Autodesk Inventor part; units mm, degrees
ref_plane "YZ Plane" through (0, 0, 0) normal (1, 0, 0) x (0, 1, 0)
ref_plane "XZ Plane" through (0, 0, 0) normal (0, 1, 0) x (-1, 0, 0)
ref_plane "XY Plane" through (0, 0, 0) normal (0, 0, 1) x (1, 0, 0)
sketch "Sketch1" plane through (0, 0, 0) normal (1, 0, 0) x (0, 1, 0)
  line L0 (0, -4.8819) -> (5, -4.8819)
  line L1 (5, -4.8819) -> (0, -4.8819)
  line L2 (0, -4.8819) -> (0, -9.8819)
  line L3 (0, -9.8819) -> (5, -9.8819)
  arc A0 (15, -4.8819) -> (5, -4.8819) centre (10, -8.1985) ccw
  arc A1 (5, -9.8819) -> (15, -9.8819) centre (10, -6.5653) ccw
  line L4 (15, -9.8819) -> (15, -4.8819)
  point P0 (0, 0)
  point P1 (0, -7.3819)
  point P2 (10, -7.3819)
  point P3 (10, -4.8819)
  point P4 (10, -9.8819)
  dimension "d0" = 5
  dimension "d1" = 10
  dimension "d2" = 5
  dimension "d3" = 5
  dimension "d4" = 10
  dimension "d5" = 6
  dimension "d6" = 6
extrude "Extrusion1" add sketch "Sketch1" along normal blind 10
sketch "Sketch7" plane through (10, 0, 0) normal (1, 0, 0) x (0, 0, -1)
  line L0 (9.8819, 15) -> (4.8819, 15)
  line L1 (9.8819, 0) -> (9.8819, 5)
  line L2 (4.8819, 0) -> (9.8819, 0)
  circle A0 centre (7.3819, 9) radius 4
  point P0 (0, 0)
  point P1 (7.3819, 15)
  point P2 (7.3819, 5)
  point P3 (9.8819, 10.0351)
  dimension "d29" = 2.5
  dimension "d30" = 10
  dimension "d31" = 4
  dimension "d33" = 5
extrude "Extrusion4" cut sketch "Sketch7" against normal blind 10
sketch "Sketch8" plane through (10, 0, 0) normal (1, 0, 0) x (0, 0, -1)
  line L0 (8.3819, 12.873) -> (8.3819, 15)
  line L1 (9.8819, 15) -> (4.8819, 15)
  line L2 (9.8819, 15) -> (4.8819, 15)
  line L3 (6.3819, 15) -> (6.3819, 12.873)
  circle A0 centre (7.3819, 9) radius 4
  line L4 (8.3819, 15) -> (6.3819, 15)
  arc A1 (8.3819, 12.873) -> (6.3819, 12.873) centre (7.3819, 9) ccw
  point P0 (0, 0)
  dimension "d36" = 1.5
  dimension "d39" = 1.5
extrude "Extrusion5" cut sketch "Sketch8" against normal blind 10 contours A0 L3 L1 L0
sketch "Sketch9" plane through (0, 0, -9.8819) normal (0, 0, -1) x (-1, 0, 0)
  circle A0 centre (-5, 13.9365) radius 0.4
  line L0 (-10, 12.873) -> (0, 12.873)
  line L1 (0, 15) -> (-10, 15)
  line L2 (-10, 15) -> (-10, 5)
  point P0 (0, 0)
  dimension "d42" = 0.8
  dimension "d43" = 1.0635
  dimension "d44" = 2.127
  dimension "d45" = 10
  dimension "d46" = 5
hole "Hole1" at (5, 13.9365, -9.8819) direction (0, 0, -1) diameter 1.5 end through all both
sketch "Sketch10" plane through (0, 0, -9.8819) normal (0, -1, 0) x (1, 0, 0)
  line L0 (12, -2) -> (12, 7)
  line L1 (12, 7) -> (-2, 7)
  line L2 (0, 7.6834) -> (10, 7.6834)
  line L3 (-2, 7) -> (-2, -2)
  line L4 (-2, -2) -> (12, -2)
  line L5 (0, -2.6834) -> (10, -2.6834)
  line L6 (0, -2.6834) -> (0, 0)
  line L7 (0, 0) -> (10, 0)
  line L8 (0, 5) -> (0, 0)
  line L9 (0, 5) -> (10, 5)
  point P0 (0, 9.8819)
  point P1 (5, 2.5)
  dimension "d54" = 14
  dimension "d56" = 2
  dimension "d57" = 2
  dimension "d58" = 5
  dimension "d59" = 2.5
  dimension "d60" = 2
  dimension "d74" = 9
extrude "Extrusion6" add sketch "Sketch10" along normal blind 1.5
sketch "Sketch11" plane through (10, 0, 0) normal (1, 0, 0) x (0, 0, -1)
  point P0 (0, 0)
sketch "Sketch12" plane through (0, -1.5, -9.8819) normal (0, -1, 0) x (1, 0, 0)
  line L0 (-2, 7) -> (-2, -2)
  line L1 (12, 7) -> (-2, 7)
  circle A0 centre (5, 2.5) radius 2.5
  point P0 (0, 9.8819)
  dimension "d63" = 7
  dimension "d64" = 4.5
  dimension "d65" = 9
  dimension "d66" = 5
hole "Hole2" at (5, -1.5, -7.3819) direction (0, 1, 0) diameter 5 depth 1.5
equation "\"d2\" = d0"
equation "\"d3\" = d0"
equation "\"d36\" = d37"
equation "\"d43\" = 0.5 * d44"
equation "\"d60\" = d57"
equation "\"d66\" = hoop_bearing_length"
equation "\"hoop_bearing_length\" = 5"
properties part number "Clamp"
The model under review builds one solid part; all positions refer to its coordinate system, in mm. A direction names the side the tool comes from. Round coordinates to 2 decimals unless told otherwise and drop trailing zeros. Order: outer loops, then holes, each group sorted by start corner. A loop starts at its lowest first (then second) coordinate and runs counter-clockwise, first axis right, second up. Notation, with made-up numbers: M -9.5,41 L 27.5,41 A27 ccw 27.5,68 Z; hole C 4.25,62.5 d10. An arc over 180 degrees is marked long. Use a Markdown table: item, result.
1) Tool access review of faces 4 (the face through (6, 14, -6.382)), 5 (the face through (10, 4, -7)), 6 (the face through (5, -1, -11.882)), 7 (the face through (0, 4, -7)): name each direction out of +Z, -Z, +X, -X, +Y, -Y from which nothing blocks a thin tool from reaching the whole face with its end or side.
Report:
| item | result |
|---|---|
| face 4 | +X, -X, +Y |
| face 5 | +Z, -Z, +X, +Y |
| face 6 | -Z, +X, -X, -Y |
| face 7 | +Z, -Z, -X, +Y |
2) Consider section A-A (y = 9). Write out the cut boundary in (x, z).
Report:
| item | result |
|---|---|
| outline | M 0,-12.48 L 10,-12.48 L 10,-11.38 L 0,-11.38 Z; M 0,-3.38 L 10,-3.38 L 10,-2.28 L 0,-2.28 Z |
3) Consider section D-D (x = 7.75). Write out the cut boundary in (y, z), then the cut area to 3 significant figures.
Report:
| item | result |
|---|---|
| outline | M -1.5,-11.88 L 0,-11.88 L 0,-9.88 L 5,-9.88 A6 ccw 15,-9.88 L 15,-8.38 L 12.87,-8.38 A4 cw long 12.87,-6.38 L 15,-6.38 L 15,-4.88 A6 ccw 5,-4.88 L 0,-4.88 L 0,-2.88 L -1.5,-2.88 Z |
| area | 71.9 mm^2 |
4) Consider section C-C (x = 5.5). Write out the cut boundary in (y, z).
Report:
| item | result |
|---|---|
| outline | M -1.5,-11.88 L 0,-11.88 L 0,-9.88 L 5,-9.88 A6 ccw 13.38,-11.52 L 13.38,-8.38 L 12.87,-8.38 A4 cw long 12.87,-6.38 L 13.38,-6.38 L 13.38,-3.24 A6 ccw 5,-4.88 L 0,-4.88 L 0,-2.88 L -1.5,-2.88 L -1.5,-4.93 L 0,-4.93 L 0,-9.83 L -1.5,-9.83 Z; M 14.5,-10.54 A6 ccw 15,-9.88 L 15,-8.38 L 14.5,-8.38 Z; M 14.5,-6.38 L 15,-6.38 L 15,-4.88 A6 ccw 14.5,-4.22 Z |
5) Consider section B-B (z = -10.75). Write out the cut boundary in (x, y), then the cut area to 3 significant figures.
Report:
| item | result |
|---|---|
| outline | M -2,-1.5 L 12,-1.5 L 12,0 L -2,0 Z; M 0,5.7 L 10,5.7 L 10,6.84 L 0,6.84 Z; M 0,11.16 L 10,11.16 L 10,14.3 L 5.66,14.3 A0.75 cw long 4.34,14.3 L 0,14.3 Z |
| area | 62.4 mm^2 |
6) Insertion check: pin 1 (1.5 mm diameter, centred on y = 2.5, z = -7, fed in from +X); pin 2 (1.1 mm diameter, centred on x = 4, y = 14, fed in from +Z); pin 3 (2 mm diameter, centred on x = 0, y = 6, fed in from -Z); pin 4 (1.4 mm diameter, centred on x = 5, y = 13.94, fed in from -Z). Each pin has a flat end and moves straight along its axis. Give the tip position at first contact, or say it passes through.
Report:
| item | result |
|---|---|
| pin 1 | x = 10 |
| pin 2 | z = -3.29 |
| pin 3 | z = -11.76 |
| pin 4 | through |
7) Draft analysis for pull direction Z (two halves, no side actions). For faces 1 (the face through (5, 2, -9.882)), 2 (the face through (5.07, 5.003, -7.22)), 3 (the face through (-2, -1, -7)), state which applies: released by +Z, released by -Z, zero draft, split by the parting line, or undercut.
Report:
| item | result |
|---|---|
| face 1 | released by -Z |
| face 2 | undercut |
| face 3 | zero draft |
8) Wall thickness on line 1 along Z through (x, y) = (5, -0.85); line 2 along Y through (x, z) = (5, -3.85); line 3 along Y through (x, z) = (8.75, -4.25): over which ranges is each line inside the solid? List them lowest first. Write a range as [from, to].
Report:
| item | result |
|---|---|
| line 1 | [-11.88, -9.88], [-4.88, -2.88] |
| line 2 | [-1.5, 0], [5.87, 7.12], [10.88, 13.19] |
| line 3 | [-1.5, 0], [5.48, 6.51], [11.49, 14.52] |
